Could you check a few things on this model? Use its own coordinates, in mm. Face numbers are marked on the shaded views. A direction names the side the tool comes from. Give positions to 0.01 mm unless a question says otherwise; leave off trailing zeros. Loops run counter-clockwise (first coordinate to the right, second up) from the corner with the lowest first, then second, coordinate; pieces in that order, holes last. Notation, with made-up numbers: (5, 43.25) -> (38, 43.25) arc R22 ccw to (38, 79.25) -> close; hole circle Ø4 at (8.25, 11). An arc over 180 degrees is marked (long way). Put each result on its own line as item: value.
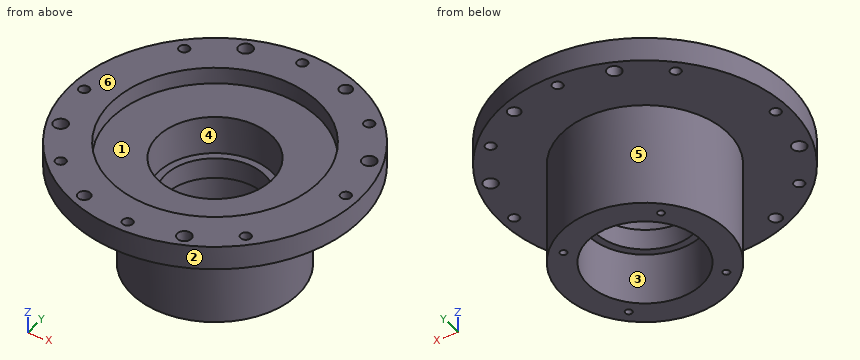
```python
from build123d import *

# Parameters (mm, degrees)
SKETCH2_R                                    = 2.5
SKETCH2_R_2                                  = 3
SKETCH2_R_3                                  = 3.4
CUT_8XM6_TIE_2XDOWEL_4XM8_MOUNT_PCD128_DEPTH = 150
SKETCH3_R                                    = 1.65
CUT_4XM4_SEAL_COVER_TAPS_DEPTH               = 10


with BuildPart() as part:
    # Sketch1 → REV_Output_Housing_Body (revolve)
    with BuildSketch(Plane(origin=(0, 0, 0), x_dir=(1, 0, 0), z_dir=(0, 1, 0))):
        Polygon((27.5, 96), (40, 96), (40, 46), (70, 46), (70, 34.5), (50, 34.5), (50, 42.5), (27.5, 42.5), (27.5, 61), (24, 61), (24, 71), (27.5, 71), align=None)
    revolve(axis=Axis((0, 0, 150), (0, 0, -1)))

    # Sketch2 → CUT_8xM6_Tie_2xDowel_4xM8_Mount_PCD128 (cut, symmetric)
    with BuildSketch(Plane.XY):
        with Locations(Location((64, 0, 0), (0, 0, 180))):
            Circle(SKETCH2_R)
        with Locations(Location((45.2548, 45.2548, 0), (0, 0, 180))):
            Circle(SKETCH2_R)
        with Locations(Location((0, 64, 0), (0, 0, 180))):
            Circle(SKETCH2_R)
        with Locations(Location((-45.2548, 45.2548, 0), (0, 0, 180))):
            Circle(SKETCH2_R)
        with Locations(Location((-64, 0, 0), (0, 0, 180))):
            Circle(SKETCH2_R)
        with Locations(Location((-45.2548, -45.2548, 0), (0, 0, 180))):
            Circle(SKETCH2_R)
        with Locations(Location((0, -64, 0), (0, 0, 180))):
            Circle(SKETCH2_R)
        with Locations(Location((45.2548, -45.2548, 0), (0, 0, 180))):
            Circle(SKETCH2_R)
        with Locations(Location((24.4917, 59.1283, 0), (0, 0, 180))):
            Circle(SKETCH2_R_2)
        with Locations(Location((-24.4917, -59.1283, 0), (0, 0, 180))):
            Circle(SKETCH2_R_2)
        with Locations(Location((59.1283, 24.4917, 0), (0, 0, 180))):
            Circle(SKETCH2_R_3)
        with Locations(Location((-24.4917, 59.1283, 0), (0, 0, 180))):
            Circle(SKETCH2_R_3)
        with Locations(Location((-59.1283, -24.4917, 0), (0, 0, 180))):
            Circle(SKETCH2_R_3)
        with Locations(Location((24.4917, -59.1283, 0), (0, 0, 180))):
            Circle(SKETCH2_R_3)
    extrude(amount=CUT_8XM6_TIE_2XDOWEL_4XM8_MOUNT_PCD128_DEPTH, both=True, mode=Mode.SUBTRACT)

    # Sketch3 → CUT_4xM4_Seal_Cover_Taps (cut)
    with BuildSketch(Plane(origin=(0, 0, -96), x_dir=(-1, 0, 0), z_dir=(0, 0, -1))):
        with Locations((23.8649, 23.8649)):
            Circle(SKETCH3_R)
        with Locations((-23.8649, 23.8649)):
            Circle(SKETCH3_R)
        with Locations((-23.8649, -23.8649)):
            Circle(SKETCH3_R)
        with Locations((23.8649, -23.8649)):
            Circle(SKETCH3_R)
    extrude(amount=-CUT_4XM4_SEAL_COVER_TAPS_DEPTH, mode=Mode.SUBTRACT)


solid = part.part
```
1. If we section it at A-A (y = 0): Count the separate pieces of the cut face and the enclosed holes in it, then the cut area to 3 significant figures.
Recorded:
separate pieces: 4
enclosed holes: 0
area: 1,820 mm^2
2. Thinking about a two-plate mould opening in Y: for the marked faces 4, 5 and 6, which applies, pulls with the +Y half, pulls with the -Y half, needs draft (parallel to the pull), parting line crosses it, or undercut?
Recorded:
face 4: undercut
face 5: parting line crosses it
face 6: needs draft
3. If we section it at C-C (x = -18): List the corners of the cut face in (y, z) for me, then the cut area to 3 significant figures.
Recorded:
outline: (-67.65, -46) -> (-35.72, -46) -> (-35.72, -96) -> (-20.79, -96) -> (-20.79, -71) -> (-15.87, -71) -> (-15.87, -61) -> (-20.79, -61) -> (-20.79, -42.5) -> (-46.65, -42.5) -> (-46.65, -34.5) -> (-67.65, -34.5) -> close; (15.87, -71) -> (20.79, -71) -> (20.79, -96) -> (35.72, -96) -> (35.72, -46) -> (67.65, -46) -> (67.65, -34.5) -> (46.65, -34.5) -> (46.65, -42.5) -> (20.79, -42.5) -> (20.79, -61) -> (15.87, -61) -> close
area: 2,260 mm^2
4. I'm going to push flat-ended pins straight in: pin 1 (2 mm diameter, centred on x = 43, y = 19.5, fed in from -Z); pin 2 (2.5 mm diameter, centred on x = -23.86, y = 23.86, fed in from -Z); pin 3 (1.5 mm diameter, centred on y = 44.5, z = -45.5, fed in from +X). Where does each tip first touch, or does it pass through?
Recorded:
pin 1: stops at z = -46
pin 2: stops at z = -86
pin 3: stops at x = 54.64
5. I need wall thicknesses on line 1 (Y direction, x = 0, z = -36); line 2 (X direction, y = 26, z = -36.5); line 3 (Z direction, x = -35, y = 29). Which ranges of each line are inside material? Lowest first, please.
Recorded:
line 1: y = -70 to -66.5, -61.5 to -50, 50 to 61.5, 66.5 to 70
line 2: x = -64.99 to -42.71, 42.71 to 56.08, 62.18 to 64.99
line 3: z = -46 to -42.5
6. If we section it at D-D (z = -76): List the corners of the cut face in (x, y) for me.
Recorded:
outline: circle Ø80 at (0, 0); hole circle Ø55 at (0, 0)
7. For the marked faces 1, 2 and 3, which set-ups out of +Z, -Z, +X, -X, +Y, -Y let a thin tool reach every point of the face, with its end or its side?
Recorded:
face 1: +Z
face 2: +Z, -Z
face 3: -Z
